Check sheet for the modelled part. Datum: model origin and axes. Units: mm. Give positions to 0.01 mm unless a question says otherwise; leave off trailing zeros. Answer in a Markdown table with one row per item. Add a question column.
(1) Thickness scan on L1, parallel to Z at x = 0.25, y = -2.5; L2, parallel to Y at x = 0, z = 2.8 (3 decimals); L3, parallel to Z at x = -1.25, y = -1.75. Record the ranges inside material, lowest first. Write a range as [from, to].
(2) Cross-section at A-A (x = -2.25). State how many separate pieces and enclosed holes the cut face has, then the cut area to 3 significant figures.
(3) Go/stop test with flat-tipped pins: pin 1 (6.5 mm diameter, centred on x = 0, y = 0, fed in from -Z); pin 2 (1.5 mm diameter, centred on x = -2, y = -1, fed in from +Z); pin 3 (2 mm diameter, centred on y = 3.5, z = 2.5, fed in from -X). Record where each tip stops, or that it passes through.
```python
from build123d import *

# Parameters (mm, degrees)
SKETCH1_R           = 2.0447
BOSS_EXTRUDE1_DEPTH = 6.35
CUT_SWEEP1_PITCH    = 1.5875
CHAMFER1_SIZE       = 0.254


with BuildPart() as part:
    # Sketch1 → Boss-Extrude1 (new body)
    with BuildSketch(Plane.XY):
        with BuildLine():
            Line((-3.01608289, 5.588), (3.01608289, 5.588))
            ThreePointArc((3.01608289, 5.588), (0, -6.35), (-3.01608289, 5.588))
        make_face()
        Circle(SKETCH1_R, mode=Mode.SUBTRACT)
    extrude(amount=BOSS_EXTRUDE1_DEPTH)

    # Cut-Sweep1: arcs per turn and ends read off the stored shape
    # Cut-Sweep1: the profile of Sketch2 profile screwed along a right-hand helix through 4.75 turns, 8 arcs to a turn; built about Z, then put on its axis
    cut_sweep1_z = Axis((0, 0, 0), (0, 0, 1))
    cut_sweep1_corners = [(2.0444, 0, -1.339811764), (3.175, 0, -0.68705955), (3.175, 0, -0.48862205), (2.0444, 0, 0.164130164)]
    with BuildLine(mode=Mode.PRIVATE) as cut_sweep1_profile:
        Line(cut_sweep1_corners[0], cut_sweep1_corners[1])
        Line(cut_sweep1_corners[1], cut_sweep1_corners[2])
        Line(cut_sweep1_corners[2], cut_sweep1_corners[3])
        Line(cut_sweep1_corners[3], cut_sweep1_corners[0])
    cut_sweep1_cap = Face(cut_sweep1_profile.wire())
    cut_sweep1_turn_angles = [0, 22.5, 45, 67.5, 90, 112.5, 135, 157.5, 180, 202.5, 225, 247.5, 270, 292.5, 315, 337.5, 360]
    cut_sweep1_turn_weights = [1, 0.9238795325112867, 1, 0.9238795325112867, 1, 0.9238795325112867, 1, 0.9238795325112867, 1, 0.9238795325112867, 1, 0.9238795325112867, 1, 0.9238795325112867, 1, 0.9238795325112867, 1]
    cut_sweep1_turn_rails = [Edge.make_bspline([Vector(p[0], p[1], 0).rotate(cut_sweep1_z, cut_sweep1_turn_angles[k]) / cut_sweep1_turn_weights[k] + Vector(0, 0, p[2] + CUT_SWEEP1_PITCH * cut_sweep1_turn_angles[k] / 360) for k in range(17)], [0, 0, 0, 1, 1, 2, 2, 3, 3, 4, 4, 5, 5, 6, 6, 7, 7, 8, 8, 8], 2, cut_sweep1_turn_weights) for p in cut_sweep1_corners]
    cut_sweep1_turn_sides = [Face.make_surface_from_curves(cut_sweep1_turn_rails[p[0]], cut_sweep1_turn_rails[p[1]]) for p in [(0, 1), (1, 2), (2, 3), (3, 0)]]
    cut_sweep1_last_angles = [1440, 1462.5, 1485, 1507.5, 1530, 1552.5, 1575, 1597.5, 1620, 1642.5, 1665, 1687.5, 1710]
    cut_sweep1_last_weights = [1, 0.9238795325112867, 1, 0.9238795325112867, 1, 0.9238795325112867, 1, 0.9238795325112867, 1, 0.9238795325112867, 1, 0.9238795325112769, 1]
    cut_sweep1_last_rails = [Edge.make_bspline([Vector(p[0], p[1], 0).rotate(cut_sweep1_z, cut_sweep1_last_angles[k]) / cut_sweep1_last_weights[k] + Vector(0, 0, p[2] + CUT_SWEEP1_PITCH * cut_sweep1_last_angles[k] / 360) for k in range(13)], [0, 0, 0, 1, 1, 2, 2, 3, 3, 4, 4, 5, 5, 6, 6, 6], 2, cut_sweep1_last_weights) for p in cut_sweep1_corners]
    cut_sweep1_last_sides = [Face.make_surface_from_curves(cut_sweep1_last_rails[p[0]], cut_sweep1_last_rails[p[1]]) for p in [(0, 1), (1, 2), (2, 3), (3, 0)]]
    cut_sweep1 = Plane(origin=(0, 0, 0), x_dir=(0.7071067811865512, 0.7071067811865438, 0), z_dir=(0, 0, 1)) * Solid(Shell([*[p.moved(Location((0, 0, CUT_SWEEP1_PITCH * i))) for i in range(4) for p in cut_sweep1_turn_sides], *cut_sweep1_last_sides, cut_sweep1_cap, cut_sweep1_cap.rotate(cut_sweep1_z, 1710).moved(Location((0, 0, CUT_SWEEP1_PITCH * 1710 / 360)))]))
    add(cut_sweep1, mode=Mode.SUBTRACT)

    # Chamfer1
    chamfer1_edges = [part.edges().sort_by_distance(p)[0] for p in [
        (0, -6.35, 0),
        (0, -6.35, 6.35),
    ]]
    chamfer(chamfer1_edges, length=CHAMFER1_SIZE)


solid = part.part
```
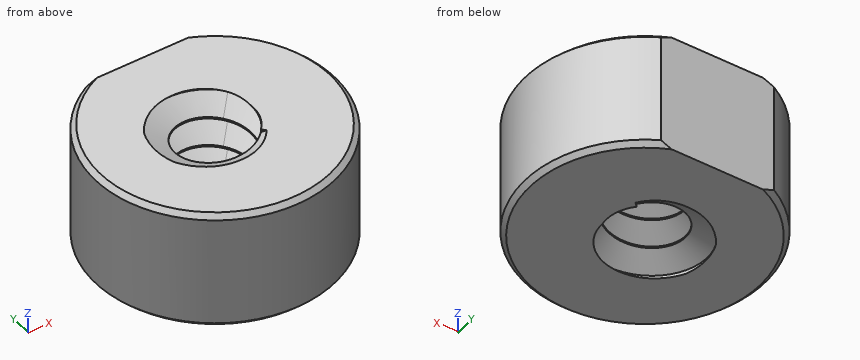
Answer below:
| question | item | result |
|---|---|---|
| 1 | L1 | z = [0.91, 1.53], [2.5, 3.12], [4.09, 4.71], [5.67, 6.3] |
| 1 | L2 | y = [-6.35, -2.045], [3.175, 5.588] |
| 1 | L3 | z = [0.94, 1.14], [2.52, 2.73], [4.11, 4.32], [5.7, 5.91] |
| 2 | separate pieces | 1 |
| 2 | enclosed holes | 3 |
| 2 | area | 57.3 mm² |
| 3 | pin 1 | stops at z = 0 |
| 3 | pin 2 | stops at z = 6.27 |
| 3 | pin 3 | stops at x = -5.84 |
